```python
from build123d import *

# Parameters (mm, degrees)
BOSS_EXTRUDE1_DEPTH = 4
SKETCH3_R           = 3.1
CUT_EXTRUDE1_DEPTH  = 1
CUT_EXTRUDE2_START  = -1
SKETCH4_R           = 3.1
CUT_EXTRUDE2_DEPTH  = 1
SKETCH5_R           = 2.4
CUT_EXTRUDE3_DEPTH  = 37.558172821
LPATTERN2_COUNT     = 5
LPATTERN2_PITCH     = 8
CUT_EXTRUDE4_DEPTH  = 36.895682192
LPATTERN3_COUNT     = 4
LPATTERN3_PITCH     = 8


with BuildPart() as part:
    # Sketch2 → Boss-Extrude1 (new, symmetric)
    with BuildSketch(Plane(origin=(0, 0, 0), x_dir=(1, 0, 0), z_dir=(0, 1, 0))):
        with BuildLine():
            Line((0, 3.5), (32, 3.5))
            ThreePointArc((32, 3.5), (35.5, 0), (32, -3.5))
            Line((32, -3.5), (0, -3.5))
            ThreePointArc((0, -3.5), (-3.5, 0), (0, 3.5))
        make_face()
    extrude(amount=BOSS_EXTRUDE1_DEPTH, both=True)

    # Sketch3 → Cut-Extrude1 (cut)
    with BuildSketch(Plane(origin=(0, 4, 0), x_dir=(1, 0, 0), z_dir=(0, 1, 0))):
        with Locations(Location((0, 0, 0), (0, 0, 270))):
            Circle(SKETCH3_R)
    cut_extrude1 = extrude(amount=-CUT_EXTRUDE1_DEPTH, mode=Mode.SUBTRACT)

    # Sketch4 → Cut-Extrude2 (cut)
    with BuildSketch(Plane(origin=(0, -4, 0), x_dir=(-1, 0, 0), z_dir=(0, -1, 0)).offset(CUT_EXTRUDE2_START)):
        with Locations(Location((0, 0, 0), (0, 0, 270))):
            Circle(SKETCH4_R)
    cut_extrude2 = extrude(amount=CUT_EXTRUDE2_DEPTH, mode=Mode.SUBTRACT)

    # Sketch5 → Cut-Extrude3 (cut, through all)
    with BuildSketch(Plane(origin=(0, -4, 0), x_dir=(-1, 0, 0), z_dir=(0, -1, 0))):
        with Locations(Location((0, 0, 0), (0, 0, 90))):
            Circle(SKETCH5_R)
    cut_extrude3 = extrude(amount=-CUT_EXTRUDE3_DEPTH, mode=Mode.SUBTRACT)

    # LPattern2: Cut-Extrude1, Cut-Extrude2, Cut-Extrude3 ×5
    with Locations(*[(i * LPATTERN2_PITCH, 0, 0) for i in range(1, LPATTERN2_COUNT)]):
        add(cut_extrude1, mode=Mode.SUBTRACT)
        add(cut_extrude2, mode=Mode.SUBTRACT)
        add(cut_extrude3, mode=Mode.SUBTRACT)

    # Sketch6 → Cut-Extrude4 (cut, symmetric)
    with BuildSketch(Plane(origin=(0, 0, 0), x_dir=(1, 0, 0), z_dir=(0, 1, 0))):
        with BuildLine():
            Line((2.814249456, 3.1), (5.185750544, 3.1))
            ThreePointArc((5.185750544, 3.1), (5.553697029, 2.856892908), (5.474391514, 2.423076923))
            ThreePointArc((5.474391514, 2.423076923), (4.5, 0), (5.474391514, -2.423076923))
            ThreePointArc((5.474391514, -2.423076923), (5.553697029, -2.856892908), (5.185750544, -3.1))
            Line((5.185750544, -3.1), (2.814249456, -3.1))
            ThreePointArc((2.814249456, -3.1), (2.446302971, -2.856892908), (2.525608486, -2.423076923))
            ThreePointArc((2.525608486, -2.423076923), (3.5, 0), (2.525608486, 2.423076923))
            ThreePointArc((2.525608486, 2.423076923), (2.446302971, 2.856892908), (2.814249456, 3.1))
        make_face()
    cut_extrude4 = extrude(amount=CUT_EXTRUDE4_DEPTH, both=True, mode=Mode.SUBTRACT)

    # LPattern3: Cut-Extrude4 ×4
    with Locations(*[(i * LPATTERN3_PITCH, 0, 0) for i in range(1, LPATTERN3_COUNT)]):
        add(cut_extrude4, mode=Mode.SUBTRACT)


solid = part.part
```
CAD build for the part. Positions are in the model's coordinates, mm. A direction names the side the tool comes from. Give positions to 0.01 mm unless a question says otherwise; leave off trailing zeros. Order: outer loops, then holes, each group sorted by start corner. A loop starts at its lowest first (then second) coordinate and runs counter-clockwise, first axis right, second up. Notation, with made-up numbers: M 41,76.25 L 89,76.25 A28 cw 89,100.25 Z; hole C 67,-22.5 d9. An arc over 180 degrees is marked long. Put each result on its own line as item: value. Start each with the question number.
(1) Saw through at A-A, the plane x = 8. Write the cut outline in (y, z), then the cut area to 3 significant figures.
(2) Which spindle directions (+Z, -Z, +X, -X, +Y, -Y) get a long thin tool onto all of the face, cutting with end or side? Do faces 1 (the cylindrical face through (27.026, -3.493, -0.672)), 2 (the cylindrical face through (3.5, 0.1, 0)), 3 (the flat face through (14, 3, 2)). Say none if no direction does.
(3) Saw through at B-B, the plane z = 0. Give the number of separate pieces and of enclosed holes in the cut face, then the cut area to 3 significant figures.
(4) Flat gauge pins, fed straight in: pin 1 Ø1.5 at (y, z) = (-2.5, 2) entering from -X; pin 2 Ø1.5 at (y, z) = (0.5, 2.5) entering from +X; pin 3 Ø2 at (x, z) = (24, -1) entering from -Y. Where does each tip first touch, or does it go through?
(5) Drill centre lines: line 1 along Z through (x, y) = (32, -3.35); line 2 along Z through (x, y) = (5, 1.5); line 3 along Z through (x, y) = (13.5, 2.75). Where is each one in solid material? Low to high.
(6) Mould opens along Z. For faces 4 (the cylindrical face through (27.5, 0.1, 0)), 5 (the flat face through (18, 4, -3)), 6 (the flat face through (16, 0, 3.5)) say: +Z half, -Z half, draft (parallel to the pull), parting line (faces both ways), or undercut.
(7) Saw through at C-C, the plane x = 31.5. Write the cut outline in (y, z), then the cut area to 3 significant figures.
Check result:
1. outline: M -4,-3.5 L 4,-3.5 L 4,-3.1 L 3,-3.1 L 3,-2.4 L -3,-2.4 L -3,-3.1 L -4,-3.1 Z; M -4,3.1 L -3,3.1 L -3,2.4 L 3,2.4 L 3,3.1 L 4,3.1 L 4,3.5 L -4,3.5 Z
1. area: 14.8 mm2
2. face 1: -Y
2. face 2: +Y, -Y
2. face 3: +Y
3. separate pieces: 10
3. enclosed holes: 0
3. area: 74.0 mm2
4. pin 1: stops at x = -3.27
4. pin 2: stops at x = 35.03
4. pin 3: passes through
5. line 1: z = -3.5 to -3.1, 3.1 to 3.5
5. line 2: z = -3.5 to -3.1, -1.8 to 1.8, 3.1 to 3.5
5. line 3: z = -3.5 to -2.95, -2.45 to 2.45, 2.95 to 3.5
6. face 4: undercut
6. face 5: draft
6. face 6: +Z half
7. outline: M -4,-3.5 L 4,-3.5 L 4,-3.06 L 3,-3.06 L 3,-2.35 L -3,-2.35 L -3,-3.06 L -4,-3.06 Z; M -4,3.06 L -3,3.06 L -3,2.35 L 3,2.35 L 3,3.06 L 4,3.06 L 4,3.5 L -4,3.5 Z
7. area: 15.6 mm2
